For this review, take the finished solid that the model builds, in its own axes (mm). A direction names the side the tool comes from. Round coordinates to 2 decimals unless told otherwise and drop trailing zeros. Loops run counter-clockwise (first coordinate to the right, second up) from the corner with the lowest first, then second, coordinate; pieces in that order, holes last. Notation, with made-up numbers: (80, 85) -> (121, 85) arc R12 cw to (121, 97) -> close; hole circle Ø7 at (85.25, 48). An arc over 180 degrees is marked (long way). Write each question's results on one line, items separated by ' | '.
```python
from build123d import *

# Parameters (mm, degrees)
SCHIZZO1_W                      = 8
SCHIZZO1_H                      = 6
ESTRUSIONE_ESTRUSIONE1_DEPTH    = 16.5
FORO_FILETTATO_M5_1_D           = 4.2
FORO_FILETTATO_M5_1_CSINK_D     = 5.05
FORO_FILETTATO_M5_1_CSINK_ANGLE = 120
SCHIZZO4_W                      = 4.25
SCHIZZO4_H                      = 1.5
TAGLIO_ESTRUSIONE1_DEPTH        = 10


with BuildPart() as part:
    # Schizzo1 → Estrusione-Estrusione1 (new body)
    with BuildSketch(Plane.XY):
        with Locations((0, 3)):
            Rectangle(SCHIZZO1_W, SCHIZZO1_H)
    extrude(amount=ESTRUSIONE_ESTRUSIONE1_DEPTH)

    # Foro filettato M5-1 (through all)
    with Locations(Plane(origin=(0, 6, 0), x_dir=(1, 0, 0), z_dir=(0, 1, 0))):
        with Locations((0, -8.25)):
            CounterSinkHole(FORO_FILETTATO_M5_1_D / 2, FORO_FILETTATO_M5_1_CSINK_D / 2, counter_sink_angle=FORO_FILETTATO_M5_1_CSINK_ANGLE)

    # Schizzo4 → Taglio-Estrusione1 (cut)
    with BuildSketch(Plane(origin=(4, 0, 0), x_dir=(0, 0, -1), z_dir=(1, 0, 0))):
        Polygon((-16.5, 0), (-16.5, 2), (-14.5, 0), align=None)
        Polygon((0, 0), (0, 2), (-2, 0), align=None)
        with Locations((-2.125, 5.25)):
            Rectangle(SCHIZZO4_W, SCHIZZO4_H)
        with Locations((-14.375, 5.25)):
            Rectangle(SCHIZZO4_W, SCHIZZO4_H)
    extrude(amount=-TAGLIO_ESTRUSIONE1_DEPTH, mode=Mode.SUBTRACT)


solid = part.part
```
1. Consider section A-A (x = 0). State the section outline as (y, z) points (3 decimals), plus the area to 3 significant figures.
Values found:
outline: (0, 2) -> (2, 0) -> (4.5, 0) -> (4.5, 4.25) -> (6, 4.25) -> (6, 5.725) -> (5.755, 6.15) -> (0, 6.15) -> close; (0, 10.35) -> (5.755, 10.35) -> (6, 10.775) -> (6, 12.25) -> (4.5, 12.25) -> (4.5, 16.5) -> (2, 16.5) -> (0, 14.5) -> close | area: 56.9 mm2
2. Consider section D-D (x = 3.25). State the section outline as (y, z) points.
Values found:
outline: (0, 2) -> (2, 0) -> (4.5, 0) -> (4.5, 4.25) -> (6, 4.25) -> (6, 12.25) -> (4.5, 12.25) -> (4.5, 16.5) -> (2, 16.5) -> (0, 14.5) -> close
3. Tool access review of faces 5 (the face through (4, 3, 8)), 6 (the face through (0, 4.5, 14)), 7 (the face through (0, 5, 4.25)): name each direction out of +Z, -Z, +X, -X, +Y, -Y from which nothing blocks a thin tool from reaching the whole face with its end or side.
Values found:
face 5: +Z, -Z, +X, +Y, -Y | face 6: +Z, +X, -X, +Y | face 7: -Z, +X, -X, +Y
4. To check wall thickness, follow probe 1 along Z at (x, y) = (0, 2.3); probe 2 along X at (y, z) = (4.45, 8.25); probe 3 along Z at (x, y) = (0, 5.7). State the ranges of each line that lie inside material, in increasing order.
Values found:
probe 1: z = 0 to 6.15, 10.35 to 16.5 | probe 2: x = -4 to -2.1, 2.1 to 4 | probe 3: z = 4.25 to 6.15, 10.35 to 12.25
5. For pin 1 (1.3 mm diameter, centred on x = 1.5, z = 14.5, fed in from +Y); pin 2 (3 mm diameter, centred on x = -0.5, z = 8, fed in from -Y), all flat-tipped, find the tip position at first contact; note any pin that passes through.
Values found:
pin 1: stops at y = 4.5 | pin 2: passes through
6. Draft analysis for pull direction Z (two halves, no side actions). For faces 1 (the face through (0.273, 2.837, 6.168)), 2 (the face through (0, 3, 0)), 3 (the face through (-2, 0, 7)), 4 (the face through (0.1, 1, 15.5)), state which applies: released by +Z, released by -Z, zero draft, split by the parting line, or undercut.
Values found:
face 1: undercut | face 2: released by -Z | face 3: zero draft | face 4: released by +Z
7. Consider section B-B (y = 3.8). State the section outline as (x, z) points.
Values found:
outline: (-4, 0) -> (4, 0) -> (4, 16.5) -> (-4, 16.5) -> close; hole circle Ø4.2 at (0, 8.25)
8. Consider section C-C (z = 8.25). State the section outline as (x, y) points (3 decimals).
Values found:
outline: (-4, 0) -> (-2.1, 0) -> (-2.1, 5.755) -> (-2.525, 6) -> (-4, 6) -> close; (2.1, 0) -> (4, 0) -> (4, 6) -> (2.525, 6) -> (2.1, 5.755) -> close
